CAD build for the part. Positions are in the model's coordinates, mm. Round coordinates to 2 decimals unless told otherwise and drop trailing zeros. Loops run counter-clockwise (first coordinate to the right, second up) from the corner with the lowest first, then second, coordinate; pieces in that order, holes last.
```python
from build123d import *

# Parameters (mm, degrees)
SKETCH_1_W      = 196
SKETCH_1_H      = 9
SKETCH_1_R      = 1.6
EXTRUDE_1_DEPTH = 3
FILLET_1_R      = 2


with BuildPart() as part:
    # 草图1 → 凸台-拉伸1 (new body)
    with BuildSketch(Plane(origin=(0, 0, 0), x_dir=(1, 0, 0), z_dir=(0, 1, 0))):
        with Locations((98, 4.5)):
            Rectangle(SKETCH_1_W, SKETCH_1_H)
        with Locations((8, 4.5)):
            Circle(SKETCH_1_R, mode=Mode.SUBTRACT)
        with Locations((28, 4.5)):
            Circle(SKETCH_1_R, mode=Mode.SUBTRACT)
        with Locations((48, 4.5)):
            Circle(SKETCH_1_R, mode=Mode.SUBTRACT)
        with Locations((68, 4.5)):
            Circle(SKETCH_1_R, mode=Mode.SUBTRACT)
        with Locations((88, 4.5)):
            Circle(SKETCH_1_R, mode=Mode.SUBTRACT)
        with Locations((108, 4.5)):
            Circle(SKETCH_1_R, mode=Mode.SUBTRACT)
        with Locations((128, 4.5)):
            Circle(SKETCH_1_R, mode=Mode.SUBTRACT)
        with Locations((148, 4.5)):
            Circle(SKETCH_1_R, mode=Mode.SUBTRACT)
        with Locations((168, 4.5)):
            Circle(SKETCH_1_R, mode=Mode.SUBTRACT)
        with Locations((188, 4.5)):
            Circle(SKETCH_1_R, mode=Mode.SUBTRACT)
    extrude(amount=EXTRUDE_1_DEPTH)

    # 圆角1
    fillet_1_edges = [part.edges().sort_by_distance(p)[0] for p in [
        (0, 1.5, -9),
        (196, 1.5, -9),
        (196, 1.5, 0),
        (0, 1.5, 0),
    ]]
    fillet(fillet_1_edges, radius=FILLET_1_R)


solid = part.part
```
Item 1: Two-plate mould, pull along Z, no slides. Class faces 1 (the flat face through (97, 1, 0)), 2 (the cylindrical face through (86.4, 1.48, -4.57)), 3 (the flat face through (97, 0, -5)): released by +Z, released by -Z, zero draft, split by the parting line, or undercut.
Answers follow:
face 1: released by +Z
face 2: undercut
face 3: zero draft
Item 2: Cut at A-A, the plane x = 48. Give the cut face in (y, z).
Answers follow:
outline: (0, -9) - (3, -9) - (3, -6.1) - (0, -6.1) - close; (0, -2.9) - (3, -2.9) - (3, 0) - (0, 0) - close
Item 3: Cut at B-B, the plane y = 0.85. State how many separate pieces and enclosed holes the cut face has, plus the area to 3 significant figures.
Answers follow:
separate pieces: 1
enclosed holes: 10
area: 1,680 mm2
Item 4: Probe line 1 (Z direction, x = 88, y = 0.8); line 2 (X direction, y = 2.5, z = -1.75); line 3 (X direction, y = 1.9, z = -8.5). List the from-to ranges inside material, lowest first.
Answers follow:
line 1: z = -9 to -6.1, -2.9 to 0
line 2: x = 0.02 to 195.98
line 3: x = 0.68 to 195.32
